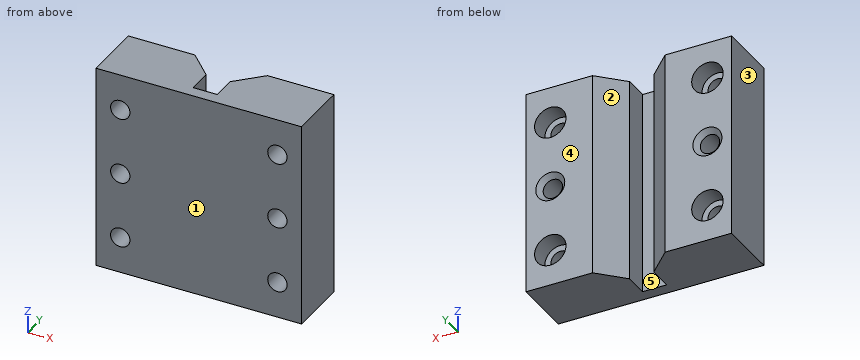
from build123d import *

# Parameters (mm, degrees)
EXTRUDE_1_DEPTH     = 42.5
SKETCH_2_R          = 6.5
CUT_EXTRUDE_1_DEPTH = 8
SKETCH_3_R          = 4
CUT_EXTRUDE_2_DEPTH = 66.096082831
CHAMFER_1_SIZE      = 2


with BuildPart() as part:
    # Эскиз1 → Бобышка-Вытянуть1 (new, symmetric)
    with BuildSketch(Plane.XY):
        Polygon((42.5, 0), (-42.5, 0), (-42.5, 25), (-15, 25), (-5, 15), (-5, 5), (5, 5), (5, 15), (15, 25), (42.5, 25), align=None)
    extrude(amount=EXTRUDE_1_DEPTH, both=True)

    # Эскиз2 → Вырез-Вытянуть1 (cut)
    with BuildSketch(Plane(origin=(0, 25, 0), x_dir=(1, 0, 0), z_dir=(0, 1, 0))):
        with Locations(Location((-32.5, 27.5, 0), (0, 0, 270))):
            Circle(SKETCH_2_R)
        with Locations(Location((-32.5, -27.5, 0), (0, 0, 270))):
            Circle(SKETCH_2_R)
        with Locations(Location((32.5, -27.5, 0), (0, 0, 270))):
            Circle(SKETCH_2_R)
        with Locations(Location((32.5, 27.5, 0), (0, 0, 270))):
            Circle(SKETCH_2_R)
    extrude(amount=-CUT_EXTRUDE_1_DEPTH, mode=Mode.SUBTRACT)

    # Эскиз3 → Вырез-Вытянуть2 (cut, through all)
    with BuildSketch(Plane(origin=(0, 25, 0), x_dir=(1, 0, 0), z_dir=(0, 1, 0))):
        with Locations(Location((-32.5, 0, 0), (0, 0, 270))):
            Circle(SKETCH_3_R)
        with Locations(Location((-32.5, 27.5, 0), (0, 0, 270))):
            Circle(SKETCH_3_R)
        with Locations(Location((32.5, 27.5, 0), (0, 0, 270))):
            Circle(SKETCH_3_R)
        with Locations(Location((32.5, 0, 0), (0, 0, 270))):
            Circle(SKETCH_3_R)
        with Locations(Location((32.5, -27.5, 0), (0, 0, 270))):
            Circle(SKETCH_3_R)
        with Locations(Location((-32.5, -27.5, 0), (0, 0, 270))):
            Circle(SKETCH_3_R)
    extrude(amount=-CUT_EXTRUDE_2_DEPTH, mode=Mode.SUBTRACT)

    # Фаска1
    chamfer_1_edges = [part.edges().sort_by_distance(p)[0] for p in [
        (-32.5, 25, -4),
        (32.5, 25, -4),
    ]]
    chamfer(chamfer_1_edges, length=CHAMFER_1_SIZE)


solid = part.part
CAD build for the part. Positions are in the model's coordinates, mm. Face numbers are marked on the shaded views. A direction names the side the tool comes from. Round coordinates to 2 decimals unless told otherwise and drop trailing zeros. Loops run counter-clockwise (first coordinate to the right, second up) from the corner with the lowest first, then second, coordinate; pieces in that order, holes last. Notation, with made-up numbers: (-18.5, 9) - (38.5, 9) arc R19 ccw to (38.5, 38) - close; hole circle Ø10 at (16, -9). An arc over 180 degrees is marked (long way). Put each result on its own line as item: value.
1. Wall check: line 1 (X direction, y = 22.5, z = 27.5); line 2 (X direction, y = 9.25, z = 1.5); line 3 (Y direction, x = 3, z = 21). Give the ranges that are in metal, low to high.
Geometry check:
line 1: -42.5 to -39, -26 to -12.5, 12.5 to 26, 39 to 42.5
line 2: -42.5 to -36.21, -28.79 to -5, 5 to 28.79, 36.21 to 42.5
line 3: 0 to 5
2. 3-axis set-ups, long thin cutter, end or side, ignore diameter. For the marked faces 1 and 2: which of +Z, -Z, +X, -X, +Y, -Y reach the whole face in a straight line?
Geometry check:
face 1: +Z, -Z, +X, -X, -Y
face 2: +Z, -Z, +Y
3. Pin check, flat tips, straight feed: P1, Ø6.5, axis at x = -30, z = -28, coming from the +Y side; P2, Ø5, axis at x = 11.5, z = 9.5, coming from the +Y side; P3, Ø3, axis at x = 1, z = -10.5, coming from the +Y side. Stop position of each tip, or through.
Geometry check:
P1: y = 17
P2: y = 24
P3: y = 5
4. Slice it at C-C on x = 32.5. List the corners of the cut face in (y, z).
Geometry check:
outline: (0, -42.5) - (25, -42.5) - (25, -34) - (17, -34) - (17, -31.5) - (0, -31.5) - close; (0, -23.5) - (17, -23.5) - (17, -21) - (25, -21) - (25, -6) - (23, -4) - (0, -4) - close; (0, 4) - (23, 4) - (25, 6) - (25, 21) - (17, 21) - (17, 23.5) - (0, 23.5) - close; (0, 31.5) - (17, 31.5) - (17, 34) - (25, 34) - (25, 42.5) - (0, 42.5) - close
5. Slice it at B-B on z = -27.5. List the corners of the cut face in (x, y), and give its area (4 significant figures).
Geometry check:
outline: (-42.5, 0) - (-36.5, 0) - (-36.5, 17) - (-39, 17) - (-39, 25) - (-42.5, 25) - close; (-28.5, 0) - (28.5, 0) - (28.5, 17) - (26, 17) - (26, 25) - (15, 25) - (5, 15) - (5, 5) - (-5, 5) - (-5, 15) - (-15, 25) - (-26, 25) - (-26, 17) - (-28.5, 17) - close; (36.5, 0) - (42.5, 0) - (42.5, 25) - (39, 25) - (39, 17) - (36.5, 17) - close
area: 1,345 mm²
6. Two-plate mould, pull along X, no slides. Class the marked faces 3, 4 and 5: released by +X, released by -X, zero draft, split by the parting line, or undercut.
Geometry check:
face 3: released by -X
face 4: zero draft
face 5: undercut
7. Slice it at A-A on y = 13.25. List the corners of the cut face in (x, z).
Geometry check:
outline: (-42.5, -42.5) - (-5, -42.5) - (-5, 42.5) - (-42.5, 42.5) - close; (5, -42.5) - (42.5, -42.5) - (42.5, 42.5) - (5, 42.5) - close; hole circle Ø8 at (-32.5, -27.5); hole circle Ø8 at (-32.5, 0); hole circle Ø8 at (-32.5, 27.5); hole circle Ø8 at (32.5, -27.5); hole circle Ø8 at (32.5, 0); hole circle Ø8 at (32.5, 27.5)
8. Slice it at D-D on y = 2.75. List the corners of the cut face in (x, z), and give its area (3 significant figures).
Geometry check:
outline: (-42.5, -42.5) - (42.5, -42.5) - (42.5, 42.5) - (-42.5, 42.5) - close; hole circle Ø8 at (-32.5, -27.5); hole circle Ø8 at (-32.5, 0); hole circle Ø8 at (-32.5, 27.5); hole circle Ø8 at (32.5, -27.5); hole circle Ø8 at (32.5, 0); hole circle Ø8 at (32.5, 27.5)
area: 6,920 mm²
